Design review of the part shown in the three views and the two pictorial views. Dimensions are in mm from the part's minimum x, y and z. A direction names the side the tool comes from. Coordinates: 2 decimals unless noted, no trailing zeros. Loops run counter-clockwise (first coordinate to the right, second up) from the corner with the lowest first, then second, coordinate; pieces in that order, holes last. Notation, with made-up numbers: M 60,64.5 L 92,64.5 A23 ccw 92,91.5 Z; hole C -11,-14 d1. An arc over 180 degrees is marked long. Put each result on its own line as item: value. Start each with the question number.
(1) Take a section at A-A, the plane x = 30. Give the boundary of the cut face in (y, z), then the cut area to 3 significant figures.
(2) The part is to be moulded in two halves that separate along X. For the marked faces 1, 2 and 3, say which applies: +X half, -X half, draft (parallel to the pull), parting line (faces both ways), or undercut.
(3) For the marked faces 4, 5 and 6, list the 3-axis set-ups (+Z, -Z, +X, -X, +Y, -Y) from which the entire face can be reached by the end or side of a thin tool; tool diameter is ignored.
(4) Take a section at B-B, the plane y = 55. Give the boundary of the cut face in (x, z).
(5) For probe 1 along Y at (x, z) = (80, 23.6); probe 2 along Y at (x, z) = (30, 13); probe 3 along Z at (x, y) = (56.5, 33), list the stretches that pass through material, from the lowest coordinate up. Write a range as [from, to].
(6) Take a section at D-D, the plane y = 8.5. Give the boundary of the cut face in (x, z), then the cut area to 3 significant figures.
(7) Clearance check with flat-ended pins moving along their axes: pin 1 (9.5 mm diameter, centred on x = 31, y = 56.5, fed in from +Z); pin 2 (10.5 mm diameter, centred on x = 47, z = 35, fed in from +Y); pin 3 (3.5 mm diameter, centred on x = 78, y = 53.5, fed in from +Z). State where each tip first meets the part, or that it passes through.
(8) Take a section at C-C, the plane z = 39. Give the boundary of the cut face in (x, y), then the cut area to 3 significant figures.
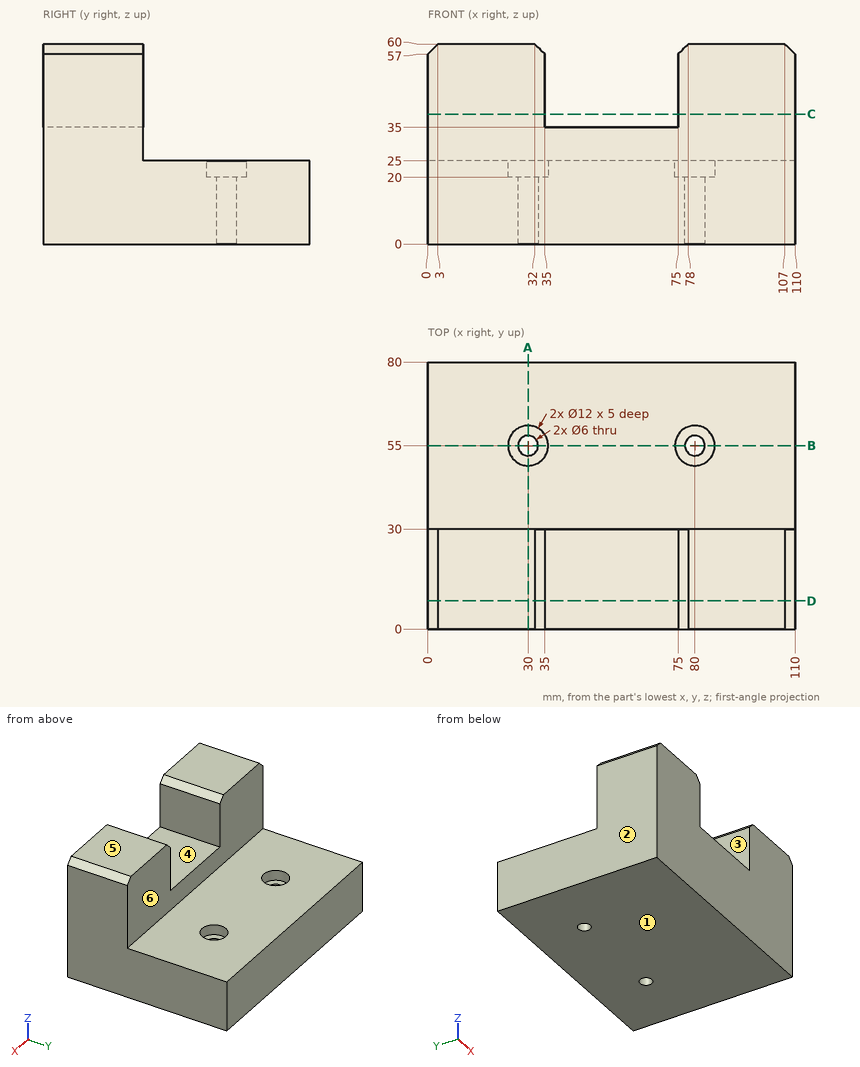
Computed values:
1. outline: M 0,0 L 52,0 L 52,20 L 49,20 L 49,25 L 30,25 L 30,60 L 0,60 Z; M 58,0 L 80,0 L 80,25 L 61,25 L 61,20 L 58,20 Z
1. area: 2,870 mm^2
2. face 1: draft
2. face 2: -X half
2. face 3: undercut
3. face 4: +Z, +Y, -Y
3. face 5: +Z, +X, -X, +Y, -Y
3. face 6: +Z, +X, -X, +Y
4. outline: M 0,0 L 27,0 L 27,20 L 24,20 L 24,25 L 0,25 Z; M 33,0 L 77,0 L 77,20 L 74,20 L 74,25 L 36,25 L 36,20 L 33,20 Z; M 83,0 L 110,0 L 110,25 L 86,25 L 86,20 L 83,20 Z
5. probe 1: y = [0, 49], [61, 80]
5. probe 2: y = [0, 52], [58, 80]
5. probe 3: z = [0, 25]
6. outline: M 0,0 L 110,0 L 110,57 L 107,60 L 78,60 L 75,57 L 75,35 L 35,35 L 35,57 L 32,60 L 3,60 L 0,57 Z
6. area: 5,580 mm^2
7. pin 1: stops at z = 25
7. pin 2: stops at y = 30
7. pin 3: stops at z = 20
8. outline: M 0,0 L 35,0 L 35,30 L 0,30 Z; M 75,0 L 110,0 L 110,30 L 75,30 Z
8. area: 2,100 mm^2
